from build123d import *

# Parameters (mm, degrees)
F0_W     = 50
F0_H     = 65
F0_R     = 1.5
F1_DEPTH = 1.5
F2_W     = 10
F2_H     = 5
F3_DEPTH = 2
F2_W_2   = 9
F2_H_2   = 10
F4_DEPTH = 5
F2_W_3   = 2
F2_W_4   = 8
F5_DEPTH = 2


with BuildPart() as f1:
    # F0 (on Top) → F1 (new body)
    with BuildSketch(Plane.XY):
        with Locations((1.260573, 11.832207)):
            Rectangle(F0_W, F0_H)
        with Locations((-21.239427, -6.667793)):
            Circle(F0_R, mode=Mode.SUBTRACT)
        with Locations((23.760573, -6.667793)):
            Circle(F0_R, mode=Mode.SUBTRACT)
        with Locations((-21.239427, 32.332207)):
            Circle(F0_R, mode=Mode.SUBTRACT)
        with Locations((23.760573, 32.332207)):
            Circle(F0_R, mode=Mode.SUBTRACT)
    extrude(amount=F1_DEPTH)

    # F2 (on face) → F3 (join)
    with BuildSketch(Plane.XY.offset(1.5)):
        with Locations((-12.739427, -5.167793)):
            Rectangle(F2_W, F2_H)
    extrude(amount=F3_DEPTH)

    # F2 (on face) → F4 (join)
    with BuildSketch(Plane.XY.offset(1.5)):
        with Locations((13.760573, 28.332207)):
            Rectangle(F2_W_2, F2_H_2)
    extrude(amount=F4_DEPTH)

    # F2 (on face) → F5 (join)
    with BuildSketch(Plane.XY.offset(1.5)):
        with Locations((19.260573, 28.332207)):
            Rectangle(F2_W_3, F2_H_2)
        with Locations((5.260573, 28.332207)):
            Rectangle(F2_W_4, F2_H_2)
    extrude(amount=F5_DEPTH)


solid = f1.part
Design review of the part built by this model. Coordinates are the model's own, in mm. A direction names the side the tool comes from. Coordinates: 2 decimals unless noted, no trailing zeros. Loops run counter-clockwise (first coordinate to the right, second up) from the corner with the lowest first, then second, coordinate; pieces in that order, holes last. Notation, with made-up numbers: (70.5, 36.5) - (117.5, 36.5) arc R27 cw to (117.5, 66.5) - close; hole circle Ø7 at (49.5, 63). An arc over 180 degrees is marked (long way). Use CSV: the item, a comma, the result in double quotes. Start each with the question number.
1. Clearance check with flat-ended pins moving along their axes: pin 1 (2 mm diameter, centred on y = 27.5, z = 2, fed in from +X); pin 2 (1.5 mm diameter, centred on x = 11.5, z = 5, fed in from +Y); pin 3 (0.6 mm diameter, centred on y = 26.5, z = 3, fed in from -X); pin 4 (2.5 mm diameter, centred on x = 15, z = 4, fed in from -Y). State where each tip first meets the part, or that it passes through.
2. Add section D-D on x = 12. Give the boundary of the cut face in (y, z).
3. Add section C-C on z = 5. Give the boundary of the cut face in (x, y).
4. Mouldability with a two-part tool opening along X and no side actions: class faces 4 (the flat face through (20.261, 28, 2)), 5 (the flat face through (-13, -7.668, 2)), 6 (the cylindrical face through (23.57, 33.82, 0.74)) as released by +X, released by -X, zero draft, split by the parting line, or undercut.
5. Add section B-B on y = 10.5. Give the boundary of the cut face in (x, z).
6. For faces 1 (the flat face through (-13, -2.668, 2)), 2 (the flat face through (19, 28, 3.5)), 3 (the flat face through (5, 28, 3.5)), list the 3-axis set-ups (+Z, -Z, +X, -X, +Y, -Y) from which the entire face can be reached by the end or side of a thin tool; tool diameter is ignored.
7. To check wall thickness, follow probe 1 along Z at (x, y) = (-5.5, 29); probe 2 along Y at (x, z) = (16.5, 6); probe 3 along Z at (x, y) = (-13, -3.5). State the ranges of each line that lie inside material, in increasing order.
8. Add section A-A on x = -15.5. Give the boundary of the cut face in (y, z).
Resolved:
1,pin 1,"x = 26.26"
1,pin 2,"y = 33.33"
1,pin 3,"x = 1.26"
1,pin 4,"y = 23.33"
2,outline,"(-20.67, 0) - (44.33, 0) - (44.33, 1.5) - (33.33, 1.5) - (33.33, 6.5) - (23.33, 6.5) - (23.33, 1.5) - (-20.67, 1.5) - close"
3,outline,"(9.26, 23.33) - (18.26, 23.33) - (18.26, 33.33) - (9.26, 33.33) - close"
4,face 4,"released by +X"
4,face 5,"zero draft"
4,face 6,"undercut"
5,outline,"(-23.74, 0) - (26.26, 0) - (26.26, 1.5) - (-23.74, 1.5) - close"
6,face 1,"+Z, +X, -X, +Y"
6,face 2,"+Z, +X, +Y, -Y"
6,face 3,"+Z, -X, +Y, -Y"
7,probe 1,"0 to 1.5"
7,probe 2,"23.33 to 33.33"
7,probe 3,"0 to 3.5"
8,outline,"(-20.67, 0) - (44.33, 0) - (44.33, 1.5) - (-2.67, 1.5) - (-2.67, 3.5) - (-7.67, 3.5) - (-7.67, 1.5) - (-20.67, 1.5) - close"
